Geometry: final body of the model. Coordinates: model frame, mm. A direction names the side the tool comes from. Give positions to 0.01 mm unless a question says otherwise; leave off trailing zeros. Loops run counter-clockwise (first coordinate to the right, second up) from the corner with the lowest first, then second, coordinate; pieces in that order, holes last.
Autodesk Inventor part; units mm, degrees
ref_plane "Work Plane1" through (30, 0, 0) normal (0, -0.5, 0.866) x (1, 0, 0)
ref_plane "YZ Plane" through (0, 0, 0) normal (1, 0, 0) x (0, 1, 0)
ref_plane "XZ Plane" through (0, 0, 0) normal (0, 1, 0) x (-1, 0, 0)
sketch "Sketch1" plane through (0, 0, 0) normal (0, 0, 1) x (1, 0, 0)
  line L0 (-0.19, 0) -> (30, 0)
  line L1 (30, 0) -> (30, 2.5)
  line L2 (30, 2.5) -> (1.6, 2.5)
  line L3 (1.6, 2.5) -> (1.1092, 2.5)
  line L4 (1.1092, 2.5) -> (0, 2.5)
  line L5 (0, 2.5) -> (0, 4.75)
  line L6 (0, 4.75) -> (-2.75, 4.75)
  line L7 (-2.75, 4.75) -> (-2.75, 1.7321)
  line L8 (-2.75, 1.7321) -> (-1.19, 1.7321)
  line L9 (-1.19, 1.7321) -> (-0.19, 0)
  line L10 (-9.3, 0) -> (36.55, 0)
  line L11 (0, -0.95) -> (0, 5.7)
  line L12 (1.6, 2.5) -> (0, 2.5) construction
  dimension "d0" = 28.4
  dimension "d1" = 0.4908
  dimension "d2" = 2.75
  dimension "d3" = 1.56
  dimension "d4" = 60
  dimension "d5" = 5
  dimension "d6" = 5
  dimension "d7" = 3.4641
  dimension "d8" = 9.5
  dimension "d19" = 30
revolve "Body" add sketch "Sketch1" angle 360 about axis through (-0.19, 0, 0) along (1, 0, 0)
sketch "Sketch2" plane through (-2.75, 0, 0) normal (-1, 0, 0) x (0, 0, 1)
  circle A0 centre (0, 0) radius 1.7321
  line L0 (0, -6.65) -> (0, 6.65)
  line L1 (-6.65, 0) -> (6.65, 0)
  line L2 (1.7321, 0) -> (0.866, -1.5)
  line L3 (0.866, -1.5) -> (-0.866, -1.5)
  line L4 (-0.866, -1.5) -> (-1.7321, 0)
  line L5 (-1.7321, 0) -> (-0.866, 1.5)
  line L6 (-0.866, 1.5) -> (0.866, 1.5)
  line L7 (0.866, 1.5) -> (1.7321, 0)
extrude "Slot" add sketch "Sketch2" against normal up to next contours L7 A0 | A0 L2 | L6 L0 A0 | A0 L0 L3 | L0 L6 A0 | A0 L3 L0 | L4 A0 | A0 L5
fillet "Fillet1" radius 2.375 1 edges at (-2.75, -4.75, 0)
thread "Thread"
chamfer "Chamfer1" distance 0.4908 distance2 0.4908 1 edges at (30, -2.5, 0) measured on face at (30, -0.5525, -0.0341)
fillet "Fillet2" radius 0.2 1 edges at (0, -2.5, 0)
ref_plane "Work Plane1" through (30, 0, 0) normal (0, -0.5, 0.866) x (1, 0, 0)
equation "\"d0\" = GEL"
equation "\"d1\" = GAL"
equation "\"d2\" = KOH"
equation "\"d3\" = INTI"
equation "\"d5\" = GD"
equation "\"d6\" = BDM"
equation "\"d7\" = 1.1547 * SW"
equation "\"d8\" = KOD"
equation "\"d19\" = NLG"
equation "\"d16\" = RR"
equation "\"d12\" = GEL"
equation "\"d14\" = -0.5 * SPD + 0.5 * GD"
equation "\"d15\" = GUL"
equation "\"d29\" = R"
equation "\"GD\" = NND"
equation "\"NLG\" = 30"
equation "\"GEL\" = 28.4"
equation "\"KOD\" = 9.5"
equation "\"KOH\" = 2.75"
equation "\"INTI\" = 1.56"
equation "\"GAL\" = 0.61345 * PTC"
equation "\"GUL\" = 0.61345 * PTC"
equation "\"BDM\" = NND"
equation "\"SW\" = 3"
equation "\"RR\" = 2.375"
equation "\"SPD\" = 4.01848"
equation "\"d28\" = R"
equation "\"R\" = 0.2"
equation "\"TOA\" = 30deg"
equation "\"THREADDIA\" = 5"
equation "\"KOD1\" = KOD - 2 * RR"
equation "\"PTC\" = 0.8"
equation "\"NND\" = 5"
equation "\"E0\" = 1.155 * SW"
equation "\"GD1\" = THREADDIA - 1.2269 * PTC"
properties part number "ANSI B18.3.4M - M5 x 0.8 x 30" material "Steel, Mild"
Item 1: Ray query, probe 1 along Z at (x, y) = (7, 2); probe 2 along X at (y, z) = (1, -1.75); probe 3 along Z at (x, y) = (5.5, -0.5). Return the intervals inside material, ascending.
Values follow:
probe 1: z = -1.5 to 1.5
probe 2: x = -2.75 to 29.99
probe 3: z = -2.45 to 2.45
Item 2: Pin query (flat end, axial travel): pin 1 (5 mm diameter, centred on x = 26.5, y = 3.5, fed in from -Z); pin 2 (4 mm diameter, centred on x = 23.5, z = -0.5, fed in from +Y); pin 3 (0.5 mm diameter, centred on x = -2, z = 0, fed in from +Y). Return the tip coordinate at first contact, or that it passes through.
Values follow:
pin 1: stops at z = -2.29
pin 2: stops at y = 2.5
pin 3: stops at y = 4.31
Item 3: Section query A-A on x = 10.5. Return loops of the section in (y, z), plus the area to 3 significant figures.
Values follow:
outline: circle Ø5 at (0, 0)
area: 19.6 mm2
Item 4: Draft query along Y for faces 1 (the face through (-2.75, -2, 0)), 2 (the face through (14.65, -0.54, 2.44)), 3 (the face through (-1.915, -0.761, -1.293)). Return one class per face: +Y half, -Y half, draft (parallel to the pull), parting line (faces both ways), or undercut.
Values follow:
face 1: draft
face 2: parting line
face 3: undercut
Item 5: Set-up query: faces 4 (the face through (30, 0, 0)), 5 (the face through (0, 2.04, -2.04)), 6 (the face through (-2, -1.5, 0)). Return all of +Z, -Z, +X, -X, +Y, -Y with unobstructed straight access to the full face (end or side cutting, diameter ignored); none if empty.
Values follow:
face 4: +Z, -Z, +X, +Y, -Y
face 5: +X
face 6: -X
